```python
from build123d import *

# Parameters (mm, degrees)
F0_W     = 600
F0_H     = 800
F1_DEPTH = 12
F2_W     = 400
F2_H     = 400
F3_DEPTH = 15
F5_R     = 3.1
F6_DEPTH = 50


with BuildPart() as f1:
    # F0 (on Top) → F1 (new body)
    with BuildSketch(Plane.XY):
        with Locations((73.317543, -274.941781)):
            Rectangle(F0_W, F0_H)
    extrude(amount=F1_DEPTH)

    # F2 (on face) → F3 (cut)
    with BuildSketch(Plane.XY.offset(12)):
        with Locations((33.317543, -274.941781)):
            Rectangle(F2_W, F2_H)
    extrude(amount=-F3_DEPTH, mode=Mode.SUBTRACT)

    # F5 (on face) → F6 (cut)
    with BuildSketch(Plane.XY.offset(12)):
        with Locations((-191.682457, -49.941781)):
            Circle(F5_R)
        with Locations((-191.682457, -499.941781)):
            Circle(F5_R)
        with Locations((258.317543, -49.941781)):
            Circle(F5_R)
        with Locations((258.317543, -499.941781)):
            Circle(F5_R)
    extrude(amount=-F6_DEPTH, mode=Mode.SUBTRACT)


solid = f1.part
```
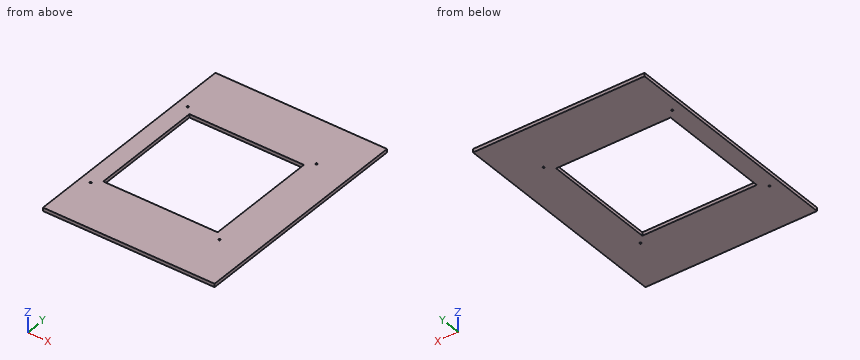
Model file for the job. Use its own axes, mm. Round coordinates to 2 decimals unless told otherwise and drop trailing zeros. Write each loop counter-clockwise with the first axis right and the second up, starting at its lowest first coordinate (ties: lowest second). Pieces come first, ordered by that corner, then holes. Notation, with made-up numbers: (42, 0.25) -> (85, 0.25) arc R18 ccw to (85, 17.25) -> close; hole circle Ø5 at (35, 33). An arc over 180 degrees is marked (long way). Answer as CSV lines item,"result".
1. Pin check, flat tips, straight feed: pin 1 Ø8 at (x, y) = (258.32, -499.94) entering from +Z; pin 2 Ø5.5 at (x, y) = (258.32, -49.94) entering from +Z. Stop position of each tip, or through.
Resolved:
pin 1,"z = 12"
pin 2,"through"
2. Drill centre lines: line 1 (Y direction, x = -192.5, z = 3.75); line 2 (Y direction, x = -49, z = 1); line 3 (X direction, y = -193, z = 3.5). Where is each one in solid material? Low to high.
Resolved:
line 1,"-674.94 to -502.93, -496.95 to -52.93, -46.95 to 125.06"
line 2,"-674.94 to -474.94, -74.94 to 125.06"
line 3,"-226.68 to -166.68, 233.32 to 373.32"
3. Slice it at C-C, the plane z = 2. List the corners of the cut face in (x, y), plus the area to 3 significant figures.
Resolved:
outline,"(-226.68, -674.94) -> (373.32, -674.94) -> (373.32, 125.06) -> (-226.68, 125.06) -> close; hole circle Ø6.2 at (-191.68, -499.94); hole circle Ø6.2 at (-191.68, -49.94); hole (-166.68, -474.94) -> (233.32, -474.94) -> (233.32, -74.94) -> (-166.68, -74.94) -> close; hole circle Ø6.2 at (258.32, -499.94); hole circle Ø6.2 at (258.32, -49.94)"
area,"320,000 mm²"
4. Slice it at B-B, the plane y = -373. List the corners of the cut face in (x, z), plus the area to 3 significant figures.
Resolved:
outline,"(-226.68, 0) -> (-166.68, 0) -> (-166.68, 12) -> (-226.68, 12) -> close; (233.32, 0) -> (373.32, 0) -> (373.32, 12) -> (233.32, 12) -> close"
area,"2,400 mm²"
5. Slice it at A-A, the plane x = 149. List the corners of the cut face in (y, z), plus the area to 3 significant figures.
Resolved:
outline,"(-674.94, 0) -> (-474.94, 0) -> (-474.94, 12) -> (-674.94, 12) -> close; (-74.94, 0) -> (125.06, 0) -> (125.06, 12) -> (-74.94, 12) -> close"
area,"4,800 mm²"
